Answer from the drawing. Dimensions are ordinates in mm from the lowest x, y and z of the part. Give positions to 0.01 mm unless a question says otherwise; leave off trailing zeros. Write each loop counter-clockwise with the first axis right and the second up, starting at its lowest first coordinate (ties: lowest second). Pieces come first, ordered by that corner, then holes.
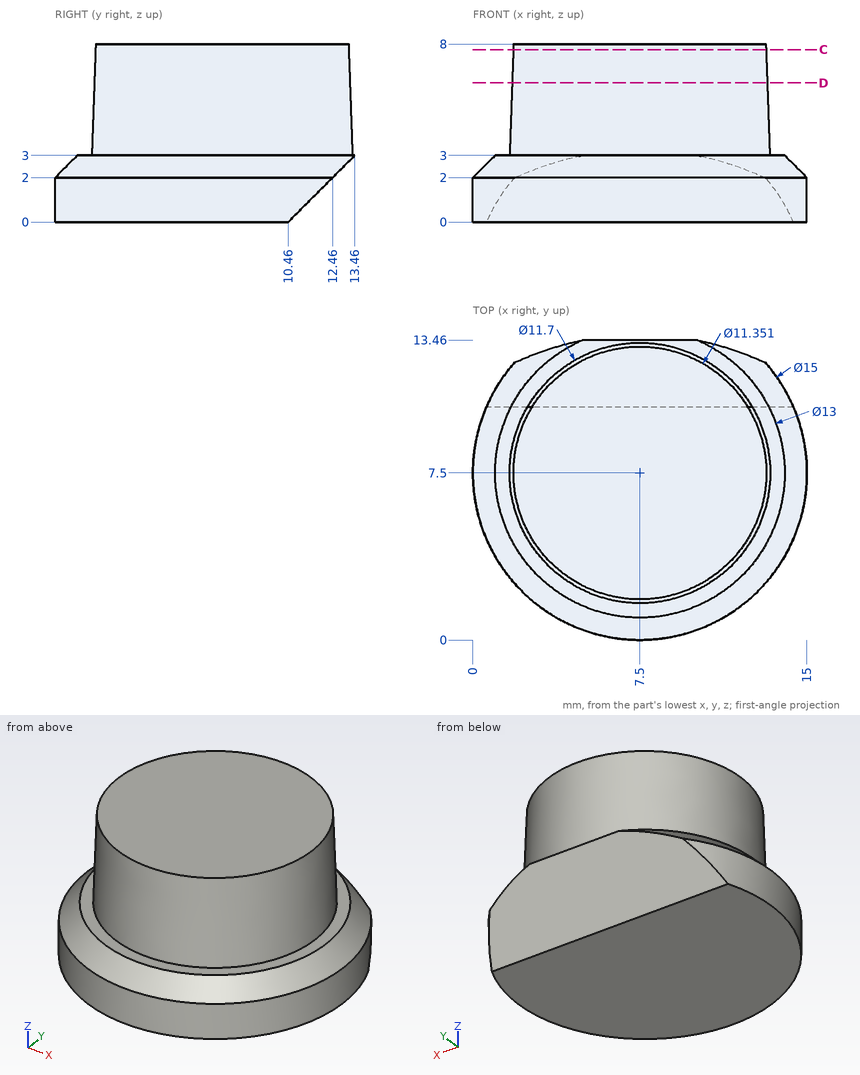
Item 1: Consider probe 1 along Z at (x, y) = (7.75, 1.5); probe 2 along X at (y, z) = (8.25, 2.25); probe 3 along X at (y, z) = (6.5, 2.5). Determine where each line is inside the solid, lowest interval first.
Conclusion:
probe 1: z = 0 to 3
probe 2: x = 0.29 to 14.71
probe 3: x = 0.57 to 14.43
Item 2: Each of these flat-tipped pins is pushed along its axis until it touches: P1, Ø3, axis at x = 13, z = 3, coming from the +Y side; P2, Ø2, axis at y = 6, z = 4.5, coming from the -X side; P3, Ø6, axis at x = 9, y = 11.5, coming from the -Z side; P4, Ø1.5, axis at x = 12.5, z = 4.5, coming from the -Y side (1 decimal). Where does it stop, or does it pass through?
Conclusion:
P1: stops at y = 13.07
P2: stops at x = 1.72
P3: stops at z = 0
P4: stops at y = 3.6
Item 3: A cutting plane is placed at D-D, the plane z = 6.25. Give the vertices of the cut face in (x, y).
Conclusion:
outline: circle Ø11.47 at (7.5, 7.5)
Item 4: A cutting plane is placed at C-C, the plane z = 7.75. Give the vertices of the cut face in (x, y).
Conclusion:
outline: circle Ø11.37 at (7.5, 7.5)
